```python
from build123d import *

# Parameters (mm, degrees)
SKETCH1_W                                  = 150
SKETCH1_H                                  = 48
BOSS_EXTRUDE1_DEPTH                        = 10
CBORE_FOR_M8_CHEESE_HEAD_SCREW1_AT_2_COUNT = 2
CBORE_FOR_M8_CHEESE_HEAD_SCREW1_AT_2_PITCH = 76
CBORE_FOR_M8_CHEESE_HEAD_SCREW1_AT_3_COUNT = 2
CBORE_FOR_M8_CHEESE_HEAD_SCREW1_AT_3_PITCH = 24
CBORE_FOR_M8_CHEESE_HEAD_SCREW1_AT_4_COUNT = 2
CBORE_FOR_M8_CHEESE_HEAD_SCREW1_AT_4_PITCH = 79.699435381
SKETCH6_R                                  = 7.5
CUT_EXTRUDE2_DEPTH                         = 5
SKETCH7_W                                  = 20
SKETCH7_H                                  = 20
CUT_EXTRUDE3_DEPTH                         = 80.37883849


with BuildPart() as part:
    # Sketch1 → Boss-Extrude1 (new body)
    with BuildSketch(Plane(origin=(0, 0, 0), x_dir=(1, 0, 0), z_dir=(0, 1, 0))):
        Rectangle(SKETCH1_W, SKETCH1_H)
    extrude(amount=BOSS_EXTRUDE1_DEPTH)

    # Sketch4 → CBORE for M8 Cheese Head Screw1 (revolve, cut)
    with BuildSketch(Plane(origin=(38, 0, 12), x_dir=(0, 0, -1), z_dir=(1, 0, 0))):
        Polygon((0, 0), (0, 12.703872786), (4.5, 10), (4.5, 5), (7.5, 5), (7.5, 0.025), (7.525, 0), align=None)
    cbore_for_m8_cheese_head_screw1 = revolve(axis=Axis((38, -6.35, 12), (0, 1, 0)), mode=Mode.SUBTRACT)

    # CBORE for M8 Cheese Head Screw1 at 2: CBORE for M8 Cheese Head Screw1 ×2
    with Locations(*[(-i * CBORE_FOR_M8_CHEESE_HEAD_SCREW1_AT_2_PITCH, 0, 0) for i in range(1, CBORE_FOR_M8_CHEESE_HEAD_SCREW1_AT_2_COUNT)]):
        add(cbore_for_m8_cheese_head_screw1, mode=Mode.SUBTRACT)

    # CBORE for M8 Cheese Head Screw1 at 3: CBORE for M8 Cheese Head Screw1 ×2
    with Locations(*[(0, 0, -i * CBORE_FOR_M8_CHEESE_HEAD_SCREW1_AT_3_PITCH) for i in range(1, CBORE_FOR_M8_CHEESE_HEAD_SCREW1_AT_3_COUNT)]):
        add(cbore_for_m8_cheese_head_screw1, mode=Mode.SUBTRACT)

    # CBORE for M8 Cheese Head Screw1 at 4: CBORE for M8 Cheese Head Screw1 ×2
    with Locations(*[Vector(-0.9535826651341417, 0, -0.3011313679370974) * (i * CBORE_FOR_M8_CHEESE_HEAD_SCREW1_AT_4_PITCH) for i in range(1, CBORE_FOR_M8_CHEESE_HEAD_SCREW1_AT_4_COUNT)]):
        add(cbore_for_m8_cheese_head_screw1, mode=Mode.SUBTRACT)

    # Sketch6 → Cut-Extrude2 (cut)
    with BuildSketch(Plane(origin=(0, 10, 0), x_dir=(1, 0, 0), z_dir=(0, 1, 0))):
        with Locations(Location((0, 0, 0), (0, 0, 270))):
            Circle(SKETCH6_R)
    extrude(amount=-CUT_EXTRUDE2_DEPTH, mode=Mode.SUBTRACT)

    # Sketch7 → Cut-Extrude3 (cut, through all)
    with BuildSketch(Plane(origin=(0, 10, 0), x_dir=(1, 0, 0), z_dir=(0, 1, 0))):
        with Locations((75, 0)):
            Rectangle(SKETCH7_W, SKETCH7_H)
        with Locations((-75, 0)):
            Rectangle(SKETCH7_W, SKETCH7_H)
    extrude(amount=-CUT_EXTRUDE3_DEPTH, mode=Mode.SUBTRACT)


solid = part.part
```
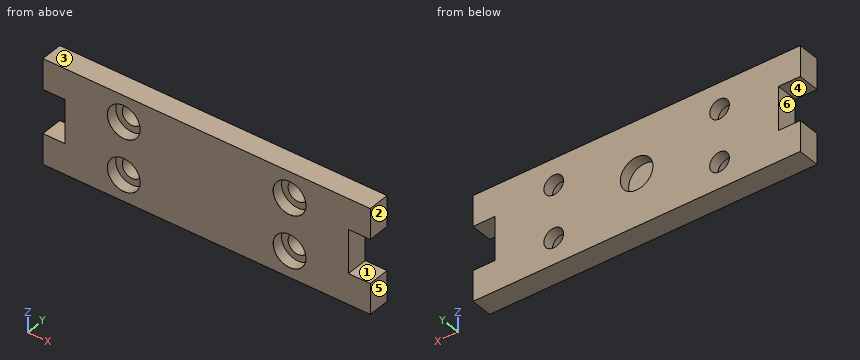
Verification items for the finished model (mm, model axes). Face numbers are marked on the shaded views. A direction names the side the tool comes from. Round coordinates to 2 decimals unless told otherwise and drop trailing zeros. Write each loop counter-clockwise with the first axis right and the second up, starting at its lowest first coordinate (ties: lowest second). Pieces come first, ordered by that corner, then holes. Notation, with made-up numbers: (73, 1) - (107, 1) arc R7 cw to (107, 8) - close; hole circle Ø9 at (14, -39). An arc over 180 degrees is marked (long way). Answer as a JSON object with one key per item and string values. Group by question number.
Q1. Thickness scan on line 1 (Z direction, x = -38, y = 6.45); line 2 (X direction, y = 6.8, z = -12); line 3 (X direction, y = 3, z = 12). Record the ranges inside material, lowest first.
Q2. Mould release check, pull along Z, two halves, no side actions. Record for the marked faces 3, 4, 5 and 6: released by +Z, released by -Z, zero draft, split by the parting line, or undercut.
Q3. Section check D-D, the plane x = 0. Enter the section's corners in (y, z), plus the area to 3 significant figures.
Q4. Section check A-A, the plane z = -12. Enter the section's corners in (x, y) (3 decimals).
Q5. Tool access check on the marked faces 1 and 2. Record the directions out of +Z, -Z, +X, -X, +Y, -Y that give a thin tool (end or side, any length) a straight path to the whole face; none if there is none.
Q6. Section check B-B, the plane x = -38. Enter the section's corners in (y, z) (3 decimals), plus the area to 3 significant figures.
Q7. Go/stop test with flat-tipped pins: pin 1 Ø4.5 at (x, z) = (-37.5, -8.5) entering from -Y; pin 2 Ø3 at (y, z) = (4.5, -0.5) entering from -X; pin 3 Ø5.5 at (x, z) = (-38, -12) entering from +Y. Record where each tip stops, or that it passes through.
Q8. Section check C-C, the plane y = 8.25. Enter the section's corners in (x, z), plus the area to 3 significant figures.
Found:
{
 "1": {"line 1": "z = -24 to -16.5, -7.5 to 7.5, 16.5 to 24", "line 2": "x = -75 to -42.5, -33.5 to 33.5, 42.5 to 75", "line 3": "x = -75 to -45.5, -30.5 to 30.5, 45.5 to 75"},
 "2": {"face 3": "released by +Z", "face 4": "undercut", "face 5": "zero draft", "face 6": "undercut"},
 "3": {"outline": "(0, -24) - (10, -24) - (10, -7.5) - (5, -7.5) - (5, 7.5) - (10, 7.5) - (10, 24) - (0, 24) - close", "area": "405 mm^2"},
 "4": {"outline": "(-75, 0) - (-45.525, 0) - (-45.5, 0.025) - (-45.5, 5) - (-42.5, 5) - (-42.5, 10) - (-75, 10) - close; (-33.5, 5) - (-30.5, 5) - (-30.5, 0.025) - (-30.475, 0) - (30.475, 0) - (30.5, 0.025) - (30.5, 5) - (33.5, 5) - (33.5, 10) - (-33.5, 10) - close; (42.5, 5) - (45.5, 5) - (45.5, 0.025) - (45.525, 0) - (75, 0) - (75, 10) - (42.5, 10) - close"},
 "5": {"face 1": "+X, +Y, -Y", "face 2": "+Z, -Z, +X, +Y, -Y"},
 "6": {"outline": "(0, -24) - (10, -24) - (10, -16.5) - (5, -16.5) - (5, -19.5) - (0.025, -19.5) - (0, -19.525) - close; (0, -4.475) - (0.025, -4.5) - (5, -4.5) - (5, -7.5) - (10, -7.5) - (10, 7.5) - (5, 7.5) - (5, 4.5) - (0.025, 4.5) - (0, 4.475) - close; (0, 19.525) - (0.025, 19.5) - (5, 19.5) - (5, 16.5) - (10, 16.5) - (10, 24) - (0, 24) - close", "area": "240 mm^2"},
 "7": {"pin 1": "stops at y = 5", "pin 2": "stops at x = -65", "pin 3": "passes through"},
 "8": {"outline": "(-75, -24) - (75, -24) - (75, -10) - (65, -10) - (65, 10) - (75, 10) - (75, 24) - (-75, 24) - (-75, 10) - (-65, 10) - (-65, -10) - (-75, -10) - close; hole circle Ø9 at (-38, -12); hole circle Ø9 at (-38, 12); hole circle Ø15 at (0, 0); hole circle Ø9 at (38, -12); hole circle Ø9 at (38, 12)", "area": "6,370 mm^2"}
}
